```python
from build123d import *

# Parameters (mm, degrees)
SKETCH_1_R               = 50
EXTRUDE_1_DEPTH          = 60
EXTRUDE_2_DEPTH          = 52
EXTRUDE_2_DEPTH_BACK     = 80
SKETCH_2_R               = 50
SKETCH_3_R               = 25
CUT_EXTRUDE_1_DEPTH      = 179.952507666
SKETCH_4_R               = 42
CUT_EXTRUDE_2_DEPTH      = 23
PATTERN_CIRCULAR_1_COUNT = 12
SKETCH_7_R               = 42.49
CUT_EXTRUDE_3_DEPTH      = 97
SKETCH_8_R               = 47.5
CUT_EXTRUDE_4_DEPTH      = 40
PATTERN_CIRCULAR_2_COUNT = 12
CUT_EXTRUDE_5_DEPTH      = 145.913767462
CUT_EXTRUDE_5_DEPTH_BACK = 145.913767462
SKETCH_12_R              = 1
CUT_EXTRUDE_8_DEPTH      = 4
SKETCH_14_R              = 0.8
CUT_EXTRUDE_9_DEPTH      = 40
SKETCH_15_R              = 0.8
CUT_EXTRUDE_10_DEPTH     = 25
PATTERN_CIRCULAR_3_COUNT = 12
SKETCH_18_R              = 42.5
CUT_EXTRUDE_11_DEPTH     = 10
SKETCH_19_R              = 14
CUT_EXTRUDE_12_DEPTH     = 10


with BuildPart() as part:
    # 草图1 → 凸台-拉伸1 (new body)
    with BuildSketch(Plane.XY):
        Circle(SKETCH_1_R)
    extrude(amount=EXTRUDE_1_DEPTH)

    # 草图2 → 凸台-拉伸2 (add, two sides: drawn at the far end of the back side and taken through both)
    with BuildSketch(Plane(origin=(0, 0, 0), x_dir=(1, 0, 0), z_dir=(0, 1, 0)).offset(-EXTRUDE_2_DEPTH_BACK)):
        with Locations(Location((0, -60, 0), (0, 0, 270))):
            Circle(SKETCH_2_R)
    extrude(amount=EXTRUDE_2_DEPTH + EXTRUDE_2_DEPTH_BACK)

    # 草图3 → 切除-拉伸1 (cut, through all)
    with BuildSketch(Plane.XZ.offset(80)):
        with Locations(Location((0, 60, 0), (0, 0, 270))):
            Circle(SKETCH_3_R)
    extrude(amount=-CUT_EXTRUDE_1_DEPTH, mode=Mode.SUBTRACT)

    # 草图4 → 切除-拉伸2 (cut)
    with BuildSketch(Plane.XZ.offset(80)):
        with Locations(Location((0, 60, 0), (0, 0, 270))):
            Circle(SKETCH_4_R)
    extrude(amount=-CUT_EXTRUDE_2_DEPTH, mode=Mode.SUBTRACT)

    # 草图5 → M3 螺纹孔1 (revolve, cut)
    with BuildSketch(Plane(origin=(0, -57, 97), x_dir=(0, 0, -1), z_dir=(1, 0, 0))):
        Polygon((0, 0), (0, 8.251075774), (1.25, 7.5), (1.25, 0), align=None)
    hole_wizard_m3_1 = revolve(axis=Axis((0, -63.35, 97), (0, 1, 0)), mode=Mode.SUBTRACT)

    # 阵列(圆周)1: M3 螺纹孔1 ×12 about axis
    pattern_circular_1_axis = Axis((0, 0, 60), (0, 1, 0))
    for i in range(1, PATTERN_CIRCULAR_1_COUNT):
        add(hole_wizard_m3_1.rotate(pattern_circular_1_axis, i * 360 / PATTERN_CIRCULAR_1_COUNT), mode=Mode.SUBTRACT)

    # 草图7 → 切除-拉伸3 (cut)
    with BuildSketch(Plane(origin=(0, 52, 0), x_dir=(1, 0, 0), z_dir=(0, 1, 0))):
        with Locations(Location((0, -60, 0), (0, 0, 270))):
            Circle(SKETCH_7_R)
    extrude(amount=-CUT_EXTRUDE_3_DEPTH, mode=Mode.SUBTRACT)

    # 草图8 → 切除-拉伸4 (cut)
    with BuildSketch(Plane(origin=(0, 52, 0), x_dir=(1, 0, 0), z_dir=(0, 1, 0))):
        with Locations(Location((0, -60, 0), (0, 0, 270))):
            Circle(SKETCH_8_R)
    extrude(amount=-CUT_EXTRUDE_4_DEPTH, mode=Mode.SUBTRACT)

    # 草图9 → M3 螺纹孔2 (revolve, cut)
    with BuildSketch(Plane(origin=(0, 12, 16), x_dir=(0, 0, 1), z_dir=(1, 0, 0))):
        Polygon((0, 0), (0, 8.251075774), (1.25, 7.5), (1.25, 0), align=None)
    hole_wizard_m3_2 = revolve(axis=Axis((0, 18.35, 16), (0, -1, 0)), mode=Mode.SUBTRACT)

    # 阵列(圆周)2: M3 螺纹孔2 ×12 about axis
    pattern_circular_2_axis = Axis((0, 0, 60), (0, 1, 0))
    for i in range(1, PATTERN_CIRCULAR_2_COUNT):
        add(hole_wizard_m3_2.rotate(pattern_circular_2_axis, i * 360 / PATTERN_CIRCULAR_2_COUNT), mode=Mode.SUBTRACT)

    # 草图11 → 切除-拉伸5 (cut, two sides: drawn at the far end of the back side and taken through both)
    with BuildSketch(Plane(origin=(0, 0, 0), x_dir=(0, 0, -1), z_dir=(1, 0, 0)).offset(-CUT_EXTRUDE_5_DEPTH_BACK)):
        Polygon((-10, 52), (-110, 52), (-110, 15.602976573), align=None)
    extrude(amount=CUT_EXTRUDE_5_DEPTH + CUT_EXTRUDE_5_DEPTH_BACK, mode=Mode.SUBTRACT)

    # 草图12 → 切除-拉伸8 (cut)
    with BuildSketch(Plane(origin=(0, 52, 0), x_dir=(-1, 0, 0), z_dir=(0, -1, 0))):
        with Locations(Location((0, -11.25, 0), (0, 0, 90))):
            Circle(SKETCH_12_R)
    extrude(amount=CUT_EXTRUDE_8_DEPTH, mode=Mode.SUBTRACT)

    # 草图14 → 切除-拉伸9 (cut)
    with BuildSketch(Plane(origin=(0, 52, 0), x_dir=(-1, 0, 0), z_dir=(0, -1, 0))):
        with Locations(Location((0, -108.75, 0), (0, 0, 90))):
            Circle(SKETCH_14_R)
    extrude(amount=CUT_EXTRUDE_9_DEPTH, mode=Mode.SUBTRACT)

    # 草图15 → 切除-拉伸10 (cut)
    with BuildSketch(Plane(origin=(0, 52, 0), x_dir=(-1, 0, 0), z_dir=(0, -1, 0))):
        with Locations(Location((48.75, -60, 0), (0, 0, 90))):
            Circle(SKETCH_15_R)
        with Locations(Location((-48.75, -60, 0), (0, 0, 90))):
            Circle(SKETCH_15_R)
    extrude(amount=CUT_EXTRUDE_10_DEPTH, mode=Mode.SUBTRACT)

    # 草图16 → M3 螺纹孔3 (revolve, cut)
    with BuildSketch(Plane(origin=(0, 46, 0), x_dir=(0, 1, 0), z_dir=(1, 0, 0))):
        Polygon((0, 0), (0, 8.251075774), (1.25, 7.5), (1.25, 0), align=None)
    hole_wizard_m3_3 = revolve(axis=Axis((0, 46, -6.35), (0, 0, 1)), mode=Mode.SUBTRACT)

    # 阵列(圆周)3: M3 螺纹孔3 ×12 about axis
    pattern_circular_3_axis = Axis((0, 0, 0), (0, 0, 1))
    for i in range(1, PATTERN_CIRCULAR_3_COUNT):
        add(hole_wizard_m3_3.rotate(pattern_circular_3_axis, i * 360 / PATTERN_CIRCULAR_3_COUNT), mode=Mode.SUBTRACT)

    # 草图18 → 切除-拉伸11 (cut)
    with BuildSketch(Plane(origin=(0, 0, 0), x_dir=(-1, 0, 0), z_dir=(0, 0, -1))):
        Circle(SKETCH_18_R)
    extrude(amount=-CUT_EXTRUDE_11_DEPTH, mode=Mode.SUBTRACT)

    # 草图19 → 切除-拉伸12 (cut)
    with BuildSketch(Plane(origin=(0, 0, 10), x_dir=(-1, 0, 0), z_dir=(0, 0, -1))):
        with Locations((-0.249858735, 28)):
            Circle(SKETCH_19_R)
    extrude(amount=-CUT_EXTRUDE_12_DEPTH, mode=Mode.SUBTRACT)


solid = part.part
```
For this review, take the finished solid that the model builds, in its own axes (mm). A direction names the side the tool comes from. Round coordinates to 2 decimals unless told otherwise and drop trailing zeros. Write each loop counter-clockwise with the first axis right and the second up, starting at its lowest first coordinate (ties: lowest second). Pieces come first, ordered by that corner, then holes. Notation, with made-up numbers: (81, -26.5) -> (87, -26.5) arc R16 ccw to (87, 2.5) -> close; hole circle Ø10 at (74, 24). An arc over 180 degrees is marked (long way). One line per question, with ' | ' between items. Start each with the question number.
(1) For line 1 along Z through (x, y) = (22, 7); line 2 along Z through (x, y) = (0, 49.1); line 3 along Z through (x, y) = (-18, -14), list the stretches that pass through material, from the lowest coordinate up. Write a range as from..to.
(2) Mouldability with a two-part tool opening along Z and no side actions: class faces 6 (the face through (33.727, -25.861, 4.93)), 7 (the face through (-18, -57, 42)), 8 (the face through (15.02, -29.59, 107.69)) as released by +Z, released by -Z, zero draft, split by the parting line, or undercut.
(3) Insertion check: P1, Ø3, axis at x = 12.5, z = 22.5, coming from the +Y side; P2, Ø3, axis at x = -38.11, z = 38, coming from the +Y side; P3, Ø1.6, axis at x = 0, z = 11.25, coming from the +Y side. Each pin has a flat end and moves straight along its axis. Give the tip position at first contact, or say it passes through.
(4) Add section B-B, the plane y = -15.5. Write out the cut boundary in (x, z).
(5) Tool access review of faces 1 (the face through (11.36, 19.48, 11.79)), 2 (the face through (-25.85, -16.1, 26.28)), 3 (the face through (-26, 34, 0)), 4 (the face through (12.62, -68.66, 19.94)), 5 (the face through (1.099, -51.084, 84.976)): name each direction out of +Z, -Z, +X, -X, +Y, -Y from which nothing blocks a thin tool from reaching the whole face with its end or side.
(6) Add section A-A, the plane z = 64. Write out the cut boundary in (x, y).
(7) Add section C-C, the plane y = -64. Write out the cut boundary in (x, z).
Answer list:
1) line 1: 10..20.64, 23.14..23.65, 96.35..96.86, 99.36..104.9 | line 2: 0..10.25, 12.25..12.5 | line 3: 10..21.51, 98.49..106.65
2) face 6: zero draft | face 7: undercut | face 8: split by the parting line
3) P1: y = -45 | P2: y = 12 | P3: y = 48
4) outline: (-47.54, 0) -> (-39.57, 0) -> (-39.57, 10) -> (39.57, 10) -> (39.57, 0) -> (47.54, 0) -> (47.54, 44.5) arc R50 ccw (long way) to (-47.54, 44.5) -> close; hole circle Ø84.98 at (0, 60)
5) face 1: -Z | face 2: +Y | face 3: -Z, +X, -X, +Y, -Y | face 4: -Y | face 5: +Y, -Y
6) outline: (-49.84, -80) -> (-41.81, -80) -> (-41.81, -57) -> (-24.68, -57) -> (-24.68, -45) -> (-42.3, -45) -> (-42.3, 12) -> (-47.33, 12) -> (-47.33, 32.35) -> (-49.84, 32.35) -> close; (24.68, -57) -> (41.81, -57) -> (41.81, -80) -> (49.84, -80) -> (49.84, 32.35) -> (47.33, 32.35) -> (47.33, 12) -> (42.3, 12) -> (42.3, -45) -> (24.68, -45) -> close
7) outline: circle Ø100 at (0, 60); hole circle Ø84 at (0, 60)
